Verification items for the finished model (mm, model axes). A direction names the side the tool comes from. Give positions to 0.01 mm unless a question says otherwise; leave off trailing zeros. Loops run counter-clockwise (first coordinate to the right, second up) from the corner with the lowest first, then second, coordinate; pieces in that order, holes last. Notation, with made-up numbers: (15.25, 16) - (20.25, 16) arc R21 cw to (20.25, 42) - close; hole circle Ø9 at (-11, -23.5). An arc over 180 degrees is marked (long way). One line per question, with ' | ' between items. Start each with the question number.
1. Thickness scan on line 1 along X through (y, z) = (2.25, -2); line 2 along Z through (x, y) = (-2, 3); line 3 along X through (y, z) = (10.75, 35). Record the ranges inside material, lowest first. Write a range as from..to.
2. Mould release check, pull along Z, two halves, no side actions. Record for faces 1 (the face through (-30, 3, -10.042)), 2 (the face through (-47.62, 9, 15)), 3 (the face through (-46, 9, 39.98)), 4 (the face through (-2.128, 2, 15)): +Z half, -Z half, draft (parallel to the pull), parting line (faces both ways), or undercut.
3. Depth check by flat-ended pin: pin 1 Ø2.5 at (x, y) = (-5, 2) entering from -Z; pin 2 Ø4 at (x, y) = (0, 3.5) entering from +Z; pin 3 Ø5.5 at (y, z) = (9.5, 3) entering from -X; pin 4 Ø4.5 at (x, z) = (-3.63, -2.03) entering from -Y. Enter the tip coordinate at first touch or a pass-through.
4. Tool access check on faces 5 (the face through (-5, 2, 9.968)), 6 (the face through (-1, 4.75, 15)), 7 (the face through (-1, 0, 15)). Record the directions out of +Z, -Z, +X, -X, +Y, -Y that give a thin tool (end or side, any length) a straight path to the whole face; none if there is none.
5. Section check D-D, the plane x = -24.5. Enter the section's corners in (y, z).
6. Section check C-C, the plane y = 3.5. State how many separate pieces and enclosed holes the cut face has, then the cut area to 3 significant figures.
from build123d import *

# Parameters (mm, degrees)
ESQUISSE2_W             = 20
ESQUISSE2_H             = 50
BOSS_EXTRU_1_DEPTH      = 4.75
ESQUISSE3_R             = 2.75
ENL_V_MAT_EXTRU_1_DEPTH = 43.183776378
ESQUISSE6_W             = 50
ESQUISSE6_H             = 6.5
BOSS_EXTRU_2_DEPTH      = 35
ESQUISSE7_W             = 3
ESQUISSE7_H             = 50
BOSS_EXTRU_3_DEPTH      = 5
ESQUISSE8_W             = 5
ESQUISSE8_H             = 10
ENL_V_MAT_EXTRU_2_DEPTH = 5.5


with BuildPart() as part:
    # Esquisse2 → Boss.-Extru.1 (new body)
    with BuildSketch(Plane(origin=(0, 0, 0), x_dir=(1, 0, 0), z_dir=(0, 1, 0))):
        with Locations((-2.628205128, -14.967948718)):
            Rectangle(ESQUISSE2_W, ESQUISSE2_H)
    extrude(amount=BOSS_EXTRU_1_DEPTH)

    # Esquisse3 → Enlèv. mat.-Extru.1 (cut, through all)
    with BuildSketch(Plane(origin=(0, 4.75, 0), x_dir=(1, 0, 0), z_dir=(0, 1, 0))):
        with Locations(Location((-3.628205128, 2.032051282, 0), (0, 0, 270))):
            Circle(ESQUISSE3_R)
        with Locations(Location((-3.628205128, -31.967948718, 0), (0, 0, 270))):
            Circle(ESQUISSE3_R)
    extrude(amount=-ENL_V_MAT_EXTRU_1_DEPTH, mode=Mode.SUBTRACT)

    # Esquisse6 → Boss.-Extru.2 (add)
    with BuildSketch(Plane.ZY.offset(12.628205128)):
        with Locations((14.958265228, 3.181677952)):
            Rectangle(ESQUISSE6_W, ESQUISSE6_H)
    extrude(amount=BOSS_EXTRU_2_DEPTH)

    # Esquisse7 → Boss.-Extru.3 (add)
    with BuildSketch(Plane(origin=(0, 6.431677952, 0), x_dir=(1, 0, 0), z_dir=(0, 1, 0))):
        with Locations((-46.119685934, -14.980159327)):
            Rectangle(ESQUISSE7_W, ESQUISSE7_H)
    extrude(amount=BOSS_EXTRU_3_DEPTH)

    # Esquisse8 → Enlèv. mat.-Extru.2 (cut)
    with BuildSketch(Plane(origin=(0, 4.75, 0), x_dir=(1, 0, 0), z_dir=(0, 1, 0))):
        with Locations((-4.628205128, -14.967948718)):
            Rectangle(ESQUISSE8_W, ESQUISSE8_H)
    extrude(amount=-ENL_V_MAT_EXTRU_2_DEPTH, mode=Mode.SUBTRACT)


solid = part.part
Results list:
1) line 1: -47.63..-6.38, -0.88..7.37 | line 2: -10.03..-4.25, 0.18..29.75, 34.18..39.97 | line 3: -47.62..-44.62
2) face 1: -Z half | face 2: draft | face 3: +Z half | face 4: undercut
3) pin 1: z = -10.03 | pin 2: z = 39.97 | pin 3: x = -47.62 | pin 4: through
4) face 5: +Y, -Y | face 6: +Z, -Z, +X, +Y | face 7: +Z, -Z, +X, -Y
5) outline: (-0.07, -10.04) - (6.43, -10.04) - (6.43, 39.96) - (-0.07, 39.96) - close
6) separate pieces: 1 | enclosed holes: 3 | area: 2,650 mm²
